The listing builds one solid part. Answer for the finished solid, in the listing's coordinates (mm). Face numbers are marked on the shaded views. Give positions to 0.01 mm unless a question says otherwise; leave off trailing zeros. Loops run counter-clockwise (first coordinate to the right, second up) from the corner with the lowest first, then second, coordinate; pieces in that order, holes last. Notation, with made-up numbers: M 3,23.5 L 21,23.5 A37 ccw 21,61.5 Z; hole C -36,-31 d6. An arc over 180 degrees is marked long. Use one line per item in the form item = value. Start each with the question number.
1. The part is cut by section B-B (z = -31.75). Write down the section's boundary in (x, y) (3 decimals).
2. Each of these flat-tipped pins is pushed along its axis until it touches: pin 1 Ø5.5 at (x, z) = (34, 4) entering from -Y; pin 2 Ø9 at (x, z) = (31.75, 31.75) entering from +Y (3 decimals); pin 3 Ø1.4 at (x, z) = (-56.15, 56.15) entering from -Y. Where does it stop, or does it pass through?
3. The mould has two halves that part along Z. Classify the marked faces 1, 2 and 3: released by +Z, released by -Z, zero draft, split by the parting line, or undercut.
4. The part is cut by section D-D (y = 1.5). Give the number of separate pieces and of enclosed holes in the cut face, and give its area (3 significant figures).
5. The part is cut by section C-C (z = 0). Write down the section's boundary in (x, y) (3 decimals).
6. The part is cut by section A-A (x = 0). Write down the section's boundary in (y, z) (3 decimals), and give its area (3 significant figures).
7. Straight lines are drawn through the part: line 1 (X direction, y = 5, z = 56.15); line 2 (X direction, y = 4.25, z = -30); line 3 (X direction, y = 7.25, z = -31.75). For each, find the intervals that lie inside material, in ascending order. Write a range as from..to.
from build123d import *

# Parameters (mm, degrees)
PLATES_DIMS_W                                    = 125
PLATES_DIMS_H                                    = 125
PLATE_THICKNESS_DEPTH                            = 9.525
F_4_40_TAPPED_HOLE1_D                            = 2.2606
LPATTERN1_COUNT                                  = 2
LPATTERN1_PITCH                                  = 112.3
LPATTERN1_COUNT_DIR2                             = 2
LPATTERN1_PITCH_DIR2                             = 112.3
FLAT_DIMS_W                                      = 19.05
FLAT_DIMS_H                                      = 19.05
FLAT_CUT_LENGTH_DEPTH                            = 4.7112
CBORE_FOR_1_4_SOCKET_HEAD_CAP_SCREW1_D           = 6.7564
CBORE_FOR_1_4_SOCKET_HEAD_CAP_SCREW1_CBORE_D     = 11.1125
CBORE_FOR_1_4_SOCKET_HEAD_CAP_SCREW1_CBORE_DEPTH = 6.35


with BuildPart() as part:
    # Plates_Dims → Plate_Thickness (new body)
    with BuildSketch(Plane(origin=(0, 0, 0), x_dir=(1, 0, 0), z_dir=(0, 1, 0))):
        Rectangle(PLATES_DIMS_W, PLATES_DIMS_H)
    extrude(amount=PLATE_THICKNESS_DEPTH)

    # #4-40 Tapped Hole1 (through all)
    with Locations(Plane(origin=(56.15, 9.525, 56.15), x_dir=(0, 0, 1), z_dir=(0, 1, 0))):
        with Locations((0, 0)):
            f_4_40_tapped_hole1 = Hole(F_4_40_TAPPED_HOLE1_D / 2)

    # LPattern1: 4-40 Tapped Hole1 2 × 2
    with Locations(*[(-j * LPATTERN1_PITCH_DIR2, 0, -i * LPATTERN1_PITCH) for i in range(LPATTERN1_COUNT) for j in range(LPATTERN1_COUNT_DIR2) if (i, j) != (0, 0)]):
        add(f_4_40_tapped_hole1, mode=Mode.SUBTRACT)

    # Cone_Cut: read off the stored shape, not the designer's step
    # Cone_Cut: loft between two sections, ruled curve by curve
    cone_cut_from = [
        Edge.make_bspline([(-28.010369629, 0, 23.684811553), (-44.140746524, 0, 16.205550811), (-51.620007265, 0, 32.335927706), (-35.489630371, 0, 39.815188447), (-19.359253476, 0, 47.294449189), (-11.879992735, 0, 31.164072294), (-28.010369629, 0, 23.684811553)], [0, 0, 0, 0, 0.5, 0.5, 0.5, 1, 1, 1, 1], 3, [1, 0.333333333, 0.333333333, 1, 0.333333333, 0.333333333, 1]),
    ]
    cone_cut_to = [
        Edge.make_bspline([(-31.396446609, 6.35, 31.396446609), (-32.103553391, 6.35, 30.689339828), (-32.810660172, 6.35, 31.396446609), (-32.103553391, 6.35, 32.103553391), (-31.396446609, 6.35, 32.810660172), (-30.689339828, 6.35, 32.103553391), (-31.396446609, 6.35, 31.396446609)], [0, 0, 0, 0, 0.5, 0.5, 0.5, 1, 1, 1, 1], 3, [1, 0.333333333, 0.333333333, 1, 0.333333333, 0.333333333, 1]),
    ]
    cone_cut = Solid(Shell([*[Face.make_surface_from_curves(cone_cut_from[k], cone_cut_to[k]) for k in range(1)], Face(Wire(cone_cut_from)), Face(Wire(cone_cut_to))]))
    add(cone_cut, mode=Mode.SUBTRACT)

    # Bottom_Groove → Groove_Cut section 0
    with BuildSketch(Plane(origin=(0, 0, 0), x_dir=(1, 0, 0), z_dir=(0, 1, 0))):
        with BuildLine():
            Line((-40.64, 43.65625), (-22.86, 43.65625))
            Line((-22.86, 43.65625), (-22.86, 19.84375))
            Line((-22.86, 19.84375), (-40.64, 19.84375))
            Line((-40.64, 19.84375), (-40.64, 43.65625))
        make_face()
    # Top_Groove → Groove_Cut section 1
    with BuildSketch(Plane(origin=(0, 6.35, 0), x_dir=(-1, 0, 0), z_dir=(0, -1, 0))):
        with BuildLine():
            Line((32.25, 43.65625), (31.25, 43.65625))
            Line((31.25, 43.65625), (31.25, 19.84375))
            Line((31.25, 19.84375), (32.25, 19.84375))
            Line((32.25, 19.84375), (32.25, 43.65625))
        make_face()
    loft(mode=Mode.SUBTRACT)

    # Flat_Dims → Flat_Cut_Length (cut)
    with BuildSketch(Plane(origin=(0, 0, 0), x_dir=(1, 0, 0), z_dir=(0, 1, 0))):
        with Locations((31.75, 0)):
            Rectangle(FLAT_DIMS_W, FLAT_DIMS_H)
    extrude(amount=FLAT_CUT_LENGTH_DEPTH, mode=Mode.SUBTRACT)

    # CBORE for 1/4 Socket Head Cap Screw1 (through all)
    with Locations(Plane(origin=(-31.75, 9.525, 0), x_dir=(0, 0, 1), z_dir=(0, 1, 0))):
        with Locations((0, 0), (31.75, 63.5), (-31.75, 63.5), (0, 31.75)):
            CounterBoreHole(CBORE_FOR_1_4_SOCKET_HEAD_CAP_SCREW1_D / 2, CBORE_FOR_1_4_SOCKET_HEAD_CAP_SCREW1_CBORE_D / 2, CBORE_FOR_1_4_SOCKET_HEAD_CAP_SCREW1_CBORE_DEPTH)


solid = part.part
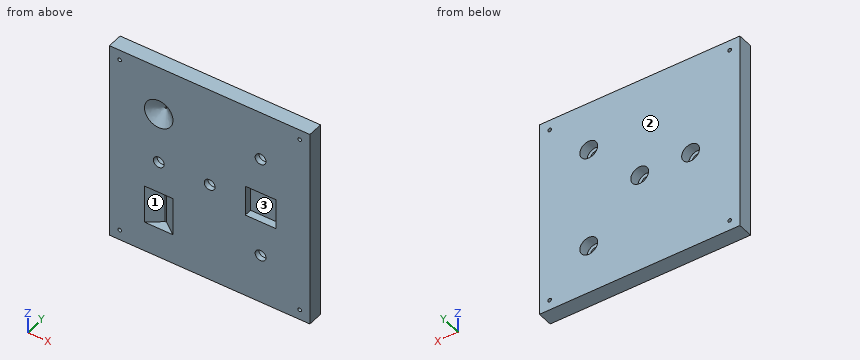
Derived:
q1.outline = M -62.5,0 L -40.64,0 L -32.25,6.35 L -31.25,6.35 L -22.86,0 L 28.372,0 L 28.372,3.175 L 26.194,3.175 L 26.194,9.525 L -62.5,9.525 Z; M 35.128,0 L 62.5,0 L 62.5,9.525 L 37.306,9.525 L 37.306,3.175 L 35.128,3.175 Z
q2.pin_1 = 4.71
q2.pin_2 = 3.175
q2.pin_3 = through
q3.face_1 = undercut
q3.face_2 = zero draft
q3.face_3 = undercut
q4.separate_pieces = 1
q4.enclosed_holes = 11
q4.area = 14,600 mm2
q5.outline = M -62.5,0 L -35.128,0 L -35.128,3.175 L -37.306,3.175 L -37.306,9.525 L -62.5,9.525 Z; M -28.372,0 L -3.378,0 L -3.378,3.175 L -5.556,3.175 L -5.556,9.525 L -26.194,9.525 L -26.194,3.175 L -28.372,3.175 Z; M 3.378,0 L 22.225,0 L 22.225,4.711 L 41.275,4.711 L 41.275,0 L 62.5,0 L 62.5,9.525 L 5.556,9.525 L 5.556,3.175 L 3.378,3.175 Z
q6.outline = M 0,-62.5 L 9.525,-62.5 L 9.525,-5.556 L 3.175,-5.556 L 3.175,-3.378 L 0,-3.378 Z; M 0,3.378 L 3.175,3.378 L 3.175,5.556 L 9.525,5.556 L 9.525,62.5 L 0,62.5 Z
q6.area = 1,100 mm2
q7.line_1 = -62.5..-57.28, -55.02..55.02, 57.28..62.5
q7.line_2 = -62.5..-35.02, -28.48..26.48, 37.02..62.5
q7.line_3 = -62.5..26.19, 37.31..62.5
